The figure shows three views and two pictorial views of one solid part (mm, origin at its lowest corner). Answer the questions. A direction names the side the tool comes from. Round coordinates to 2 decimals unless told otherwise and drop trailing zeros. Order: outer loops, then holes, each group sorted by start corner. A loop starts at its lowest first (then second) coordinate and runs counter-clockwise, first axis right, second up. Notation, with made-up numbers: (-32.75, 83) - (-24.75, 83) arc R33 cw to (-24.75, 113) - close; hole circle Ø4 at (39.5, -16.75). An arc over 180 degrees is marked (long way). One line per question, with ' | ' between items. Start each with the question number.
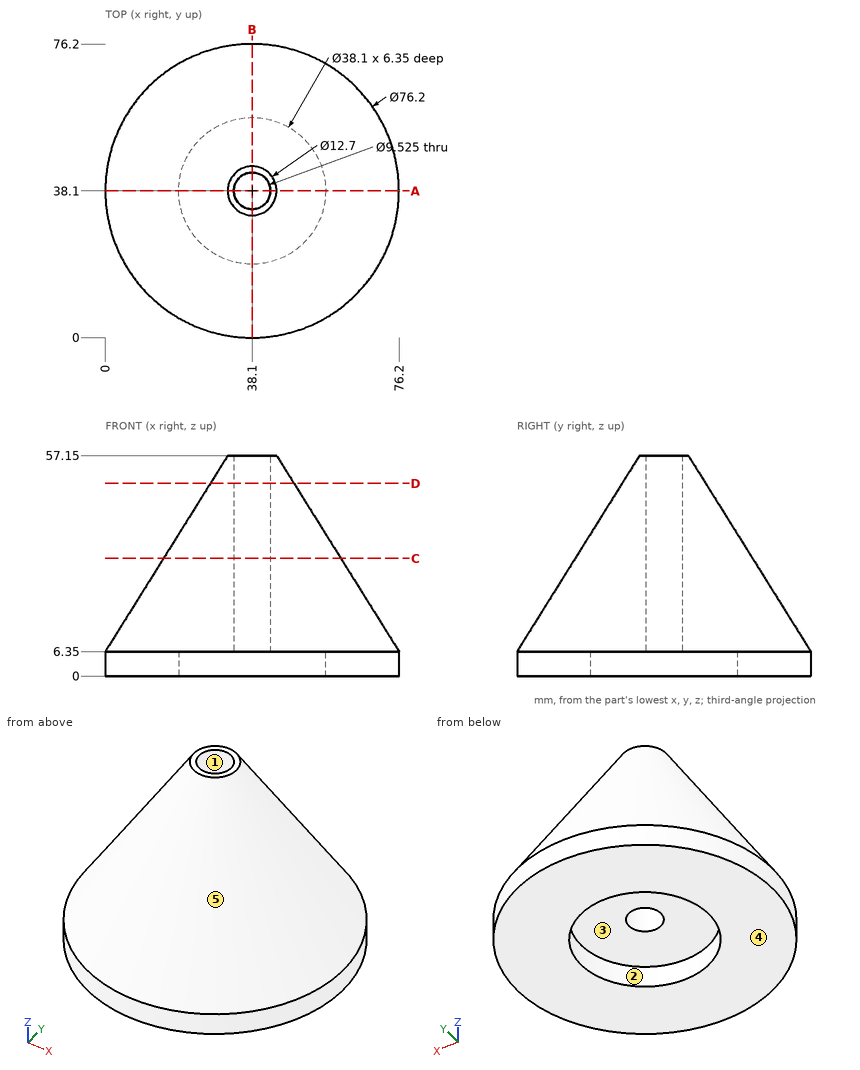
1) Section A-A on y = 38.1 is taken. Give the vertices of the cut face in (x, z).
2) Section C-C on z = 30.5 is taken. Give the vertices of the cut face in (x, y) (1 decimal), and give its area (3 significant figures).
3) Determine the mould class of the marked faces 3, 4 and 5 for opening direction Y: released by +Y, released by -Y, zero draft, split by the parting line, or undercut.
4) For the marked faces 1 and 2, determine the directions among +Z, -Z, +X, -X, +Y, -Y from which every point of the face is accessible in a straight line to the end or side of a thin tool.
5) Straight lines are drawn through the part: line 1 (Y direction, x = 38.1, z = 2.75); line 2 (Y direction, x = 42, z = 53). For each, find the intervals that lie inside material, in ascending order.
6) Flat-ended cylindrical pins translate along their axes: pin 1 (2 mm diameter, centred on y = 39.5, z = 16.5, fed in from +X); pin 2 (2 mm diameter, centred on x = 59, y = 24.5, fed in from +Z); pin 3 (2 mm diameter, centred on x = 50, y = 56, fed in from -Z); pin 4 (10 mm diameter, centred on x = 49, y = 68, fed in from +Z). Find the tip coordinate at first contact, or state that the pin passes through.
7) Section D-D on z = 50 is taken. Give the vertices of the cut face in (x, y) (1 decimal).
Recorded:
1) outline: (0, 0) - (19.05, 0) - (19.05, 6.35) - (33.34, 6.35) - (33.34, 57.15) - (31.75, 57.15) - (0, 6.35) - close; (42.86, 6.35) - (57.15, 6.35) - (57.15, 0) - (76.2, 0) - (76.2, 6.35) - (44.45, 57.15) - (42.86, 57.15) - close
2) outline: circle Ø46 at (38.1, 38.1); hole circle Ø9.5 at (38.1, 38.1) | area: 1,590 mm²
3) face 3: undercut | face 4: zero draft | face 5: split by the parting line
4) face 1: +Z, -Z | face 2: -Z
5) line 1: y = 0 to 19.05, 57.15 to 76.2 | line 2: y = 30.05 to 35.37, 40.83 to 46.15
6) pin 1: stops at x = 70.45 | pin 2: stops at z = 29.01 | pin 3: stops at z = 0 | pin 4: stops at z = 24.39
7) outline: circle Ø21.6 at (38.1, 38.1); hole circle Ø9.5 at (38.1, 38.1)
